from build123d import *
from OCP.BRepFilletAPI import BRepFilletAPI_MakeChamfer

# Parameters (mm, degrees)
SKETCH_1_R          = 12
SKETCH_1_R_2        = 0.5
EXTRUDE_1_DEPTH     = 1.18
SKETCH_2_R          = 0.5
EXTRUDE_2_DEPTH     = 2
SKETCH_3_R          = 1
CUT_EXTRUDE_1_DEPTH = 0.6
CHAMFER_1_SIZE      = 0.5
CHAMFER_1_SIZE2     = 0.500055206
SKETCH_4_R          = 2.4
CUT_EXTRUDE_2_DEPTH = 4.6
FILLET_1_R          = 0.1


with BuildPart() as part:
    # 草图1 → 凸台-拉伸1 (new body)
    with BuildSketch(Plane(origin=(0, 0, 0), x_dir=(1, 0, 0), z_dir=(0, 1, 0))):
        with Locations(Location((0, 0, 0), (0, 0, 270))):
            Circle(SKETCH_1_R)
        with Locations(Location((-9.4, 0, 0), (0, 0, 270))):
            Circle(SKETCH_1_R_2, mode=Mode.SUBTRACT)
        with Locations(Location((-6.62, 0, 0), (0, 0, 270))):
            Circle(SKETCH_1_R_2, mode=Mode.SUBTRACT)
        with Locations(Location((0, 9.4, 0), (0, 0, 270))):
            Circle(SKETCH_1_R_2, mode=Mode.SUBTRACT)
        with Locations(Location((0, 6.62, 0), (0, 0, 270))):
            Circle(SKETCH_1_R_2, mode=Mode.SUBTRACT)
        with Locations(Location((9.4, 0, 0), (0, 0, 270))):
            Circle(SKETCH_1_R_2, mode=Mode.SUBTRACT)
        with Locations(Location((6.62, 0, 0), (0, 0, 270))):
            Circle(SKETCH_1_R_2, mode=Mode.SUBTRACT)
        with Locations(Location((0, -9.4, 0), (0, 0, 270))):
            Circle(SKETCH_1_R_2, mode=Mode.SUBTRACT)
        with Locations(Location((0, -6.62, 0), (0, 0, 270))):
            Circle(SKETCH_1_R_2, mode=Mode.SUBTRACT)
    extrude(amount=EXTRUDE_1_DEPTH)

    # 草图2 → 凸台-拉伸2 (add)
    # profile 1 of 4: a face of its own
    with BuildSketch(Plane(origin=(0, 1.18, 0), x_dir=(1, 0, 0), z_dir=(0, 1, 0))):
        with BuildLine():
            Line((-2.828427125, 0), (-9.780813828, 6.952386703))
            ThreePointArc((-9.780813828, 6.952386703), (-12, 0), (-9.780813828, -6.952386703))
            Line((-9.780813828, -6.952386703), (-2.828427125, 0))
        make_face()
        with Locations(Location((-9.4, 0, 0), (0, 0, 270))):
            Circle(SKETCH_2_R, mode=Mode.SUBTRACT)
        with Locations(Location((-6.62, 0, 0), (0, 0, 270))):
            Circle(SKETCH_2_R, mode=Mode.SUBTRACT)
    # profile 2 of 4: a face of its own
    with BuildSketch(Plane(origin=(0, 1.18, 0), x_dir=(1, 0, 0), z_dir=(0, 1, 0))):
        with BuildLine():
            Line((-6.952386703, 9.780813828), (0, 2.828427125))
            Line((0, 2.828427125), (6.952386703, 9.780813828))
            ThreePointArc((6.952386703, 9.780813828), (0, 12), (-6.952386703, 9.780813828))
        make_face()
        with Locations(Location((0, 6.62, 0), (0, 0, 270))):
            Circle(SKETCH_2_R, mode=Mode.SUBTRACT)
        with Locations(Location((0, 9.4, 0), (0, 0, 270))):
            Circle(SKETCH_2_R, mode=Mode.SUBTRACT)
    # profile 3 of 4: a face of its own
    with BuildSketch(Plane(origin=(0, 1.18, 0), x_dir=(1, 0, 0), z_dir=(0, 1, 0))):
        with BuildLine():
            ThreePointArc((12, 0), (11.431748902, 3.648988495), (9.780813828, 6.952386703))
            Line((9.780813828, 6.952386703), (2.828427125, 0))
            Line((2.828427125, 0), (9.780813828, -6.952386703))
            ThreePointArc((9.780813828, -6.952386703), (11.431748902, -3.648988495), (12, 0))
        make_face()
        with Locations(Location((6.62, 0, 0), (0, 0, 270))):
            Circle(SKETCH_2_R, mode=Mode.SUBTRACT)
        with Locations(Location((9.4, 0, 0), (0, 0, 270))):
            Circle(SKETCH_2_R, mode=Mode.SUBTRACT)
    # profile 4 of 4: a face of its own
    with BuildSketch(Plane(origin=(0, 1.18, 0), x_dir=(1, 0, 0), z_dir=(0, 1, 0))):
        with BuildLine():
            Line((0.000156121, -2.828271004), (-6.952386703, -9.780813828))
            ThreePointArc((-6.952386703, -9.780813828), (0.000662371, -11.999999982), (6.953466414, -9.780046259))
            Line((6.953466414, -9.780046259), (0.000156121, -2.828271004))
        make_face()
        with Locations(Location((0, -9.4, 0), (0, 0, 270))):
            Circle(SKETCH_2_R, mode=Mode.SUBTRACT)
        with Locations(Location((0, -6.62, 0), (0, 0, 270))):
            Circle(SKETCH_2_R, mode=Mode.SUBTRACT)
    extrude(amount=EXTRUDE_2_DEPTH)

    # 草图3 → 切除-拉伸1 (cut)
    with BuildSketch(Plane(origin=(0, 3.18, 0), x_dir=(1, 0, 0), z_dir=(0, 1, 0))):
        with Locations(Location((-9.4, 0, 0), (0, 0, 270))):
            Circle(SKETCH_3_R)
        with Locations(Location((-6.62, 0, 0), (0, 0, 270))):
            Circle(SKETCH_3_R)
        with Locations(Location((0, 9.4, 0), (0, 0, 270))):
            Circle(SKETCH_3_R)
        with Locations(Location((0, 6.62, 0), (0, 0, 270))):
            Circle(SKETCH_3_R)
        with Locations(Location((9.4, 0, 0), (0, 0, 270))):
            Circle(SKETCH_3_R)
        with Locations(Location((6.62, 0, 0), (0, 0, 270))):
            Circle(SKETCH_3_R)
        with Locations(Location((0, -9.4, 0), (0, 0, 270))):
            Circle(SKETCH_3_R)
        with Locations(Location((0, -6.62, 0), (0, 0, 270))):
            Circle(SKETCH_3_R)
    extrude(amount=-CUT_EXTRUDE_1_DEPTH, mode=Mode.SUBTRACT)

    # 倒角1: one chamfer whose edges measure the first distance from different faces: ONE call of the kernel's chamfer builder (chamfer() names one face for all edges)
    chamfer_1_edges_1 = [part.edges().sort_by_distance(p)[0] for p in [
        (-6.304620476, 3.18, 3.476193351),
        (-2.828427125, 2.18, 0),
        (-6.304620476, 3.18, -3.476193351),
        (-3.476193351, 3.18, -6.304620476),
        (0, 2.18, -2.828427125),
        (3.476193351, 3.18, -6.304620476),
        (6.304620476, 3.18, -3.476193351),
        (2.828427125, 2.18, 0),
        (6.304620476, 3.18, 3.476193351),
        (3.476811268, 3.18, 6.304158631),
        (-3.476115291, 3.18, 6.304542416),
    ]]
    chamfer_1_edges_2 = [part.edges().sort_by_distance(p)[0] for p in [
        (0.000156121, 2.18, 2.828271004),
    ]]
    chamfer_1_side_2 = [part.faces().sort_by_distance(p)[0] for p in [
        (-3.476115291, 2.18, 6.304542416),
    ]]
    chamfer_1 = BRepFilletAPI_MakeChamfer(part.part.solid().wrapped)
    for e in chamfer_1_edges_1:
        chamfer_1.Add(CHAMFER_1_SIZE, e.wrapped)
    for e in chamfer_1_edges_2:
        chamfer_1.Add(CHAMFER_1_SIZE, CHAMFER_1_SIZE2, e.wrapped, chamfer_1_side_2[0].wrapped)  # the first distance lies on this face
    add(Compound.cast(chamfer_1.Shape()), mode=Mode.REPLACE)

    # 草图4 → 切除-拉伸2 (cut)
    with BuildSketch(Plane(origin=(0, 1.18, 0), x_dir=(1, 0, 0), z_dir=(0, 1, 0))):
        with Locations(Location((0, 0, 0), (0, 0, 270))):
            Circle(SKETCH_4_R)
    extrude(amount=-CUT_EXTRUDE_2_DEPTH, mode=Mode.SUBTRACT)

    # 圆角1
    fillet_1_edges = [part.edges().sort_by_distance(p)[0] for p in [
        (0, 0, -2.4),
        (0, 1.18, -2.4),
    ]]
    fillet(fillet_1_edges, radius=FILLET_1_R)


solid = part.part
Verification items for the finished model (mm, model axes). A direction names the side the tool comes from. Coordinates: 2 decimals unless noted, no trailing zeros. Loops run counter-clockwise (first coordinate to the right, second up) from the corner with the lowest first, then second, coordinate; pieces in that order, holes last. Notation, with made-up numbers: (-12.5, 30.25) -> (32.5, 30.25) arc R17 ccw to (32.5, 38.25) -> close; hole circle Ø3 at (-9.5, 34). An arc over 180 degrees is marked (long way). Answer as a JSON object with one key per item and string values. Group by question number.
Item 1: Sectioned sample at C-C on z = -9.4. Record the boundary of the cut face in (x, y), plus the area to 3 significant figures.
Item 2: Sectioned sample at D-D on x = 9.4. Record the boundary of the cut face in (y, z), plus the area to 3 significant figures.
Item 3: Scan lines: probe 1 along X at (y, z) = (0.3, 0); probe 2 along Z at (x, y) = (0, 1.95). Record each from-to range of solid material in increasing order.
Item 4: Sectioned sample at A-A on y = 2.3. State how many separate pieces and enclosed holes the cut face has, plus the area to 3 significant figures.
Item 5: Depth check by flat-ended pin: pin 1 (1.6 mm diameter, centred on x = -6.5, z = 0, fed in from +Y); pin 2 (1.5 mm diameter, centred on y = 2, z = -5, fed in from +X). Enter the tip coordinate at first touch or a pass-through.
Item 6: Tool access check on faces 1 (the cylindrical face through (-0.192, 1.272, 7.082)), 2 (the cylindrical face through (0, 2.9, 8.4)). Record the directions out of +Z, -Z, +X, -X, +Y, -Y that give a thin tool (end or side, any length) a straight path to the whole face; none if there is none.
Evaluation:
{
 "1": {"outline": "(-7.46, 0) -> (-0.5, 0) -> (-0.5, 2.58) -> (-1, 2.58) -> (-1, 3.18) -> (-5.86, 3.18) -> (-6.57, 2.68) -> (-6.57, 1.18) -> (-7.46, 1.18) -> close; (0.5, 0) -> (7.46, 0) -> (7.46, 1.18) -> (6.57, 1.18) -> (6.57, 2.68) -> (5.86, 3.18) -> (1, 3.18) -> (1, 2.58) -> (0.5, 2.58) -> close", "area": "39.8 mm²"},
 "2": {"outline": "(0, -7.46) -> (1.18, -7.46) -> (1.18, -6.57) -> (2.68, -6.57) -> (3.18, -5.86) -> (3.18, -1) -> (2.58, -1) -> (2.58, -0.5) -> (0, -0.5) -> close; (0, 0.5) -> (2.58, 0.5) -> (2.58, 1) -> (3.18, 1) -> (3.18, 5.86) -> (2.68, 6.57) -> (1.18, 6.57) -> (1.18, 7.46) -> (0, 7.46) -> close", "area": "39.8 mm²"},
 "3": {"probe 1": "x = -12 to -9.9, -8.9 to -7.12, -6.12 to -2.4, 2.4 to 6.12, 7.12 to 8.9, 9.9 to 12", "probe 2": "z = -12 to -9.9, -8.9 to -7.12, -6.12 to -3.18, 3.18 to 6.12, 7.12 to 8.9, 9.9 to 12"},
 "4": {"separate pieces": "4", "enclosed holes": "8", "area": "271 mm²"},
 "5": {"pin 1": "stops at y = 2.58", "pin 2": "stops at x = 11.22"},
 "6": {"face 1": "+Y, -Y", "face 2": "+Y"}
}
